Geometry: final body of the model. Coordinates: model frame, mm. A direction names the side the tool comes from. Give positions to 0.01 mm unless a question says otherwise; leave off trailing zeros. Write each loop counter-clockwise with the first axis right and the second up, starting at its lowest first coordinate (ties: lowest second). Pieces come first, ordered by that corner, then holes.
Q1. Cut plane A-A on x = 0. Return the cut outline in (y, z).
Q2. Cut plane D-D on y = -7. Return the cut outline in (x, z), plus the area to 3 significant figures.
Q3. Pin query (flat end, axial travel): pin 1 (3 mm diameter, centred on x = -14.5, z = 28.5, fed in from +Y); pin 2 (5.5 mm diameter, centred on x = -17.5, y = 3.5, fed in from -Z); pin 3 (3 mm diameter, centred on x = -15, z = 28, fed in from -Y); pin 4 (8.5 mm diameter, centred on x = 0, y = 0, fed in from -Z). Return the tip coordinate at first contact, or that it passes through.
Q4. Cut plane C-C on z = 27.25. Return the cut outline in (x, y).
Q5. Reachability of faces 4 (the face through (-16, 8, 28)), 5 (the face through (16, 8, 28)), 6 (the face through (16, 0, 28)) from +Z, -Z, +X, -X, +Y, -Y: full face, straight path, thin tool, end or side. Return the list, or none.
Q6. Draft query along X for faces 1 (the face through (19.5, 4, 28)), 2 (the face through (0, -12.5, 15)), 3 (the face through (0, 11.5, 15)). Return one class per face: pulls with the +X half, pulls with the -X half, needs draft (parallel to the pull), parting line crosses it, or undercut.
Q7. Line query: L1, parallel to Y at x = 0, z = 0.4; L2, parallel to Y at x = -10.5, z = 3.5. Output: solid intervals per line, ascending.
Q8. Cut plane B-B on z = 10.75. Return the cut outline in (x, y), plus the area to 3 significant figures.
```python
from build123d import *

# Parameters (mm, degrees)
SKETCH1_W           = 25
SKETCH1_H           = 25
BOSS_EXTRUDE2_DEPTH = 30
SHELL3_T            = -1
SKETCH4_R           = 5.25
CUT_EXTRUDE2_DEPTH  = 25
SKETCH5_W           = 7
SKETCH5_H           = 8
BOSS_EXTRUDE3_DEPTH = 4
SKETCH6_R           = 1.75
CUT_EXTRUDE3_DEPTH  = 10


with BuildPart() as part:
    # Sketch1 → Boss-Extrude2 (new body)
    with BuildSketch(Plane.XY):
        Rectangle(SKETCH1_W, SKETCH1_H)
    extrude(amount=BOSS_EXTRUDE2_DEPTH)

    # Shell3
    shell3_openings = [part.faces().sort_by_distance(p)[0] for p in [
        (0, 0, 30),
    ]]
    offset(amount=SHELL3_T, openings=shell3_openings, kind=Kind.INTERSECTION)

    # Sketch4 → Cut-Extrude2 (cut)
    with BuildSketch(Plane(origin=(0, 0, 0), x_dir=(-1, 0, 0), z_dir=(0, 0, -1))):
        Circle(SKETCH4_R)
    extrude(amount=-CUT_EXTRUDE2_DEPTH, mode=Mode.SUBTRACT)

    # Sketch5 → Boss-Extrude3 (add)
    with BuildSketch(Plane.XY.offset(30)):
        with Locations((16, 4)):
            Rectangle(SKETCH5_W, SKETCH5_H)
        with Locations((-16, 4)):
            Rectangle(SKETCH5_W, SKETCH5_H)
    extrude(amount=-BOSS_EXTRUDE3_DEPTH)

    # Sketch6 → Cut-Extrude3 (cut)
    with BuildSketch(Plane.XY.offset(30)):
        with Locations((15.682122387, 4.043264387)):
            Circle(SKETCH6_R)
        with Locations((-16.367627776, 4.043264387)):
            Circle(SKETCH6_R)
    extrude(amount=-CUT_EXTRUDE3_DEPTH, mode=Mode.SUBTRACT)


solid = part.part
```
Data:
1. outline: (-12.5, 0) - (-5.25, 0) - (-5.25, 1) - (-11.5, 1) - (-11.5, 30) - (-12.5, 30) - close; (5.25, 0) - (12.5, 0) - (12.5, 30) - (11.5, 30) - (11.5, 1) - (5.25, 1) - close
2. outline: (-12.5, 0) - (12.5, 0) - (12.5, 30) - (11.5, 30) - (11.5, 1) - (-11.5, 1) - (-11.5, 30) - (-12.5, 30) - close
2. area: 83.0 mm2
3. pin 1: stops at y = 8
3. pin 2: stops at z = 26
3. pin 3: stops at y = 0
3. pin 4: passes through
4. outline: (-19.5, 0) - (-12.5, 0) - (-12.5, -12.5) - (12.5, -12.5) - (12.5, 0) - (19.5, 0) - (19.5, 8) - (12.5, 8) - (12.5, 12.5) - (-12.5, 12.5) - (-12.5, 8) - (-19.5, 8) - close; hole circle Ø3.5 at (-16.37, 4.04); hole (-11.5, -11.5) - (11.5, -11.5) - (11.5, 11.5) - (-11.5, 11.5) - close; hole circle Ø3.5 at (15.68, 4.04)
5. face 4: +Z, -Z, -X, +Y
5. face 5: +Z, -Z, +X, +Y
5. face 6: +Z, -Z, +X, -Y
6. face 1: pulls with the +X half
6. face 2: needs draft
6. face 3: undercut
7. L1: y = -12.5 to -5.25, 5.25 to 12.5
7. L2: y = -12.5 to -11.5, 11.5 to 12.5
8. outline: (-12.5, -12.5) - (12.5, -12.5) - (12.5, 12.5) - (-12.5, 12.5) - close; hole (-11.5, -11.5) - (11.5, -11.5) - (11.5, 11.5) - (-11.5, 11.5) - close
8. area: 96.0 mm2
